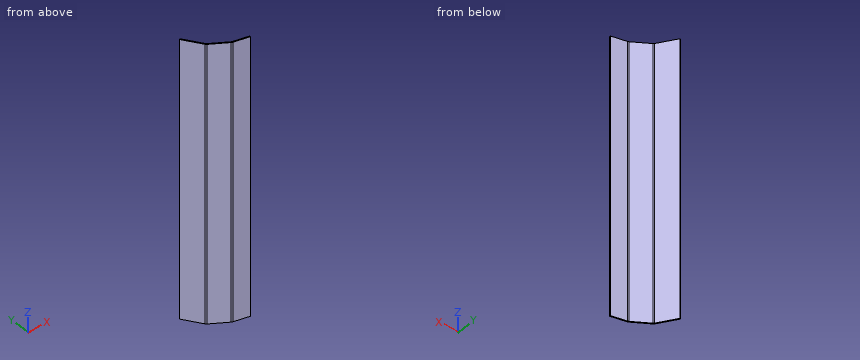
```python
from build123d import *

# Parameters (mm, degrees)
NESTED_SUPPORT_SKIN_BEHIND_TOE_DEPTH = 272


with BuildPart() as part:
    # Nested support skin behind toe profile → Nested support skin behind toe (new body)
    with BuildSketch(Plane.XY):
        with BuildLine():
            Line((135.5, 3.091362383), (121.100256736, 6.681621613))
            ThreePointArc((121.100256736, 6.681621613), (120.605812494, 6.851872419), (120.148443712, 7.105396074))
            Line((120.148443712, 7.105396074), (104.793241848, 17.462610509))
            ThreePointArc((104.793241848, 17.462610509), (104.312801158, 17.865748115), (103.92667627, 18.359965434))
            Line((103.92667627, 18.359965434), (93.151951904, 35.603128879))
            Line((93.151951904, 35.603128879), (92.303903808, 35.073209614))
            Line((92.303903808, 35.073209614), (103.078628174, 17.83004617))
            ThreePointArc((103.078628174, 17.83004617), (103.593461357, 17.171089745), (104.234048945, 16.633572937))
            Line((104.234048945, 16.633572937), (119.589250809, 6.276358502))
            ThreePointArc((119.589250809, 6.276358502), (120.19907585, 5.938326962), (120.85833484, 5.711325887))
            Line((120.85833484, 5.711325887), (135.5, 2.060748754))
            Line((135.5, 2.060748754), (135.5, 3.091362383))
        make_face()
    extrude(amount=NESTED_SUPPORT_SKIN_BEHIND_TOE_DEPTH)


solid = part.part
```
The model under review builds one solid part; all positions refer to its coordinate system, in mm. Coordinates: 2 decimals unless noted, no trailing zeros. Order: outer loops, then holes, each group sorted by start corner. A loop starts at its lowest first (then second) coordinate and runs counter-clockwise, first axis right, second up. Notation, with made-up numbers: (35.25, -29.5) -> (63.25, -29.5) arc R9 cw to (63.25, -24.5) -> close; hole circle Ø5 at (43, 23.5). An arc over 180 degrees is marked (long way). Answer in a Markdown table with one row per item. Add a question column.
Item 1: We need section C-C on y = 12.5. Write out the cut boundary in (x, z), plus the area to 3 significant figures.
Item 2: Clearance check with flat-ended pins moving along their axes: pin 1 (2 mm diameter, centred on y = 30.5, z = 51.5, fed in from -X); pin 2 (2 mm diameter, centred on x = 110, z = 125, fed in from -Y); pin 3 (12 mm diameter, centred on x = 108.5, z = 128.5, fed in from -Y). State where each tip first meets the part, or that it passes through.
Item 3: We need section A-A on z = 130. Write out the cut boundary in (x, y), plus the area to 3 significant figures.
Item 4: To check wall thickness, follow probe 1 along Y at (x, z) = (121, 22.5); probe 2 along Y at (x, z) = (102, 73.5); probe 3 along X at (y, z) = (24.5, 240.5). State the ranges of each line that lie inside material, in increasing order.
Item 5: We need section B-B on x = 111. Write out the cut boundary in (y, z).
Final values:
| question | item | result |
|---|---|---|
| 1 | outline | (110.36, 0) -> (112.15, 0) -> (112.15, 272) -> (110.36, 272) -> close |
| 1 | area | 486 mm2 |
| 2 | pin 1 | stops at x = 94.54 |
| 2 | pin 2 | stops at y = 12.07 |
| 2 | pin 3 | stops at y = 9.71 |
| 3 | outline | (92.3, 35.07) -> (103.08, 17.83) arc R4 ccw to (104.23, 16.63) -> (119.59, 6.28) arc R4 ccw to (120.86, 5.71) -> (135.5, 2.06) -> (135.5, 3.09) -> (121.1, 6.68) arc R3 cw to (120.15, 7.11) -> (104.79, 17.46) arc R3 cw to (103.93, 18.36) -> (93.15, 35.6) -> close |
| 3 | area | 56.5 mm2 |
| 4 | probe 1 | y = 5.68 to 6.71 |
| 4 | probe 2 | y = 19.56 to 21.44 |
| 4 | probe 3 | x = 98.91 to 100.09 |
| 5 | outline | (12.07, 0) -> (13.28, 0) -> (13.28, 272) -> (12.07, 272) -> close |
